Geometry: final body of the model. Coordinates: model frame, mm. A direction names the side the tool comes from. Coordinates: 2 decimals unless noted, no trailing zeros. Loops run counter-clockwise (first coordinate to the right, second up) from the corner with the lowest first, then second, coordinate; pieces in that order, holes last. Notation, with made-up numbers: M 5.5,-6.5 L 11.5,-6.5 A27 ccw 11.5,18.5 Z; hole C -24,7 d4. An arc over 180 degrees is marked long. Write item = value, one per line. Start each with the question number.
```python
from build123d import *

# Parameters (mm, degrees)
SKETCH_1_W          = 42
SKETCH_1_H          = 42
SKETCH_1_R          = 1.6
SKETCH_1_R_2        = 11
EXTRUDE_1_DEPTH     = 3
FILLET_1_R          = 5
SKETCH_2_R          = 18
SKETCH_2_R_2        = 16
EXTRUDE_2_DEPTH     = 7
SKETCH_3_R          = 13
CUT_EXTRUDE_1_DEPTH = 3


with BuildPart() as part:
    # 草图1 → 凸台-拉伸1 (new body)
    with BuildSketch(Plane.XY):
        Rectangle(SKETCH_1_W, SKETCH_1_H)
        with Locations((-15.5, 15.5)):
            Circle(SKETCH_1_R, mode=Mode.SUBTRACT)
        with Locations((15.5, 15.5)):
            Circle(SKETCH_1_R, mode=Mode.SUBTRACT)
        with Locations((15.5, -15.5)):
            Circle(SKETCH_1_R, mode=Mode.SUBTRACT)
        with Locations((-15.5, -15.5)):
            Circle(SKETCH_1_R, mode=Mode.SUBTRACT)
        Circle(SKETCH_1_R_2, mode=Mode.SUBTRACT)
    extrude(amount=EXTRUDE_1_DEPTH)

    # 圆角1
    fillet_1_edges = [part.edges().sort_by_distance(p)[0] for p in [
        (-21, -21, 1.5),
        (-21, 21, 1.5),
        (21, 21, 1.5),
        (21, -21, 1.5),
    ]]
    fillet(fillet_1_edges, radius=FILLET_1_R)

    # 草图2 → 凸台-拉伸2 (add)
    with BuildSketch(Plane(origin=(0, 0, 0), x_dir=(-1, 0, 0), z_dir=(0, 0, -1))):
        with Locations(Location((0, 0, 0), (0, 0, 180))):
            Circle(SKETCH_2_R)
        Circle(SKETCH_2_R_2, mode=Mode.SUBTRACT)
    extrude(amount=EXTRUDE_2_DEPTH)

    # 草图3 → 切除-拉伸1 (cut)
    with BuildSketch(Plane(origin=(0, 0, 0), x_dir=(-1, 0, 0), z_dir=(0, 0, -1))):
        Circle(SKETCH_3_R)
    extrude(amount=-CUT_EXTRUDE_1_DEPTH, mode=Mode.SUBTRACT)


solid = part.part
```
Item 1: Section query B-B (x = 12). Return the cut outline in (y, z).
Item 2: Section query C-C (y = 5). Return the cut outline in (x, z).
Item 3: Line query: line 1 (Y direction, x = 15.5, z = 1.55); line 2 (Z direction, x = 10.5, y = 10); line 3 (Y direction, x = 0, z = -4.5). Output: solid intervals per line, ascending. Write a range as from..to.
Item 4: Reachability of faces 1 (the flat face through (-12, 11, -7)), 2 (the cylindrical face through (-13.267, -12.165, -3.451)) from +Z, -Z, +X, -X, +Y, -Y: full face, straight path, thin tool, end or side. Return the list, or none.
Item 5: First-contact query: pin 1 (1.5 mm diameter, centred on x = -10.5, z = -5.5, fed in from +Y); pin 2 (3.5 mm diameter, centred on x = -15.5, y = 15.5, fed in from -Z); pin 3 (1.5 mm diameter, centred on y = -7.5, z = -4, fed in from +X). Flat tips, straight axial feed; report the tip coordinate or a pass-through.
Item 6: Section query D-D (x = -15.5). Return the cut outline in (y, z), plus the area to 3 significant figures.
Item 7: Pull-direction query (Y, two-part tool) for faces 3 (the cylindrical face through (3.47, -15.62, -3.45)), 4 (the flat face through (0, -21, 1)), 5 (the flat face through (-10, 10, 3)); classes: released by +Y, released by -Y, zero draft, split by the parting line, or undercut.
Item 8: Section query A-A (z = 0.75). Return the cut outline in (x, y), plus the area to 3 significant figures.
Verdict:
q1.outline = M -21,0 L -13.42,0 L -13.42,-7 L -10.58,-7 L -10.58,0 L -5,0 L -5,3 L -21,3 Z; M 5,0 L 10.58,0 L 10.58,-7 L 13.42,-7 L 13.42,0 L 21,0 L 21,3 L 5,3 Z
q2.outline = M -21,0 L -17.29,0 L -17.29,-7 L -15.2,-7 L -15.2,0 L -12,0 L -12,3 L -21,3 Z; M 12,0 L 15.2,0 L 15.2,-7 L 17.29,-7 L 17.29,0 L 21,0 L 21,3 L 12,3 Z
q3.line_1 = -21..-17.1, -13.9..13.9, 17.1..21
q3.line_2 = 0..3
q3.line_3 = -18..-16, 16..18
q4.face_1 = -Z, +X, -X, +Y, -Y
q4.face_2 = -Z
q5.pin_1 = 15.13
q5.pin_2 = 0
q5.pin_3 = 16.69
q6.outline = M -21,0 L -17.1,0 L -17.1,3 L -21,3 Z; M -13.9,0 L -9.15,0 L -9.15,-7 L -3.97,-7 L -3.97,0 L 3.97,0 L 3.97,-7 L 9.15,-7 L 9.15,0 L 13.9,0 L 13.9,3 L -13.9,3 Z; M 17.1,0 L 21,0 L 21,3 L 17.1,3 Z
q6.area = 179 mm2
q7.face_3 = undercut
q7.face_4 = released by -Y
q7.face_5 = zero draft
q8.outline = M -21,-16 A5 ccw -16,-21 L 16,-21 A5 ccw 21,-16 L 21,16 A5 ccw 16,21 L -16,21 A5 ccw -21,16 Z; hole C -15.5,-15.5 d3.2; hole C -15.5,15.5 d3.2; hole C 0,0 d26; hole C 15.5,-15.5 d3.2; hole C 15.5,15.5 d3.2
q8.area = 1,180 mm2
